```python
from build123d import *

# Parameters (mm, degrees)
SKETCH1_W           = 38
SKETCH1_H           = 53
SKETCH1_W_2         = 22
SKETCH1_H_2         = 42
BOSS_EXTRUDE1_DEPTH = 20
SKETCH2_W           = 8
SKETCH2_H           = 20
BOSS_EXTRUDE2_DEPTH = 20
SKETCH3_R           = 2.75
SKETCH3_R_2         = 1.6
CUT_EXTRUDE1_DEPTH  = 3
SKETCH3_2_R         = 1.6
CUT_EXTRUDE2_DEPTH  = 57.588426379
SKETCH4_R           = 1.6
CUT_EXTRUDE3_DEPTH  = 52.606685613
BOSS_EXTRUDE3_DEPTH = 8
FILLET2_R           = 3
FILLET1_R           = 5


with BuildPart() as part:
    # Sketch1 → Boss-Extrude1 (new body)
    with BuildSketch(Plane.XY):
        Rectangle(SKETCH1_W, SKETCH1_H)
        Rectangle(SKETCH1_W_2, SKETCH1_H_2, mode=Mode.SUBTRACT)
    extrude(amount=BOSS_EXTRUDE1_DEPTH)

    # Sketch2 → Boss-Extrude2 (add)
    with BuildSketch(Plane.XY.offset(20)):
        with Locations((-15, 11.5)):
            Rectangle(SKETCH2_W, SKETCH2_H)
    extrude(amount=BOSS_EXTRUDE2_DEPTH)

    # Sketch3 → Cut-Extrude1 (cut)
    # profile 1 of 2: a face of its own
    with BuildSketch(Plane(origin=(-11, 0, 0), x_dir=(0, 0, -1), z_dir=(1, 0, 0))):
        with Locations((-36, 11.5)):
            Circle(SKETCH3_R)
        with Locations((-36, 11.5)):
            Circle(SKETCH3_R_2, mode=Mode.SUBTRACT)
    # profile 2 of 2: a face of its own
    with BuildSketch(Plane(origin=(-11, 0, 0), x_dir=(0, 0, -1), z_dir=(1, 0, 0))):
        with Locations((-28, 11.5)):
            Circle(SKETCH3_R)
        with Locations((-28, 11.5)):
            Circle(SKETCH3_R_2, mode=Mode.SUBTRACT)
    extrude(amount=-CUT_EXTRUDE1_DEPTH, mode=Mode.SUBTRACT)

    # Sketch3<2> → Cut-Extrude2 (cut, through all)
    with BuildSketch(Plane(origin=(-11, 0, 0), x_dir=(0, 0, -1), z_dir=(1, 0, 0))):
        with Locations((-36, 11.5)):
            Circle(SKETCH3_2_R)
        with Locations((-28, 11.5)):
            Circle(SKETCH3_2_R)
    extrude(amount=-CUT_EXTRUDE2_DEPTH, mode=Mode.SUBTRACT)

    # Sketch4 → Cut-Extrude3 (cut, through all)
    with BuildSketch(Plane(origin=(0, 0, 0), x_dir=(-1, 0, 0), z_dir=(0, 0, -1))):
        with Locations((-5.1, -23.9)):
            Circle(SKETCH4_R)
        with Locations((5.1, -23.9)):
            Circle(SKETCH4_R)
        with Locations((-5.1, 23.9)):
            Circle(SKETCH4_R)
        with Locations((5.1, 23.9)):
            Circle(SKETCH4_R)
    extrude(amount=-CUT_EXTRUDE3_DEPTH, mode=Mode.SUBTRACT)

    # Sketch5 → Boss-Extrude3 (add)
    with BuildSketch(Plane.ZY.offset(19)):
        Polygon((32, 1.5), (20, -3.5), (20, 1.5), align=None)
        Polygon((20, 26.5), (20, 21.5), (32, 21.5), align=None)
    extrude(amount=-BOSS_EXTRUDE3_DEPTH)

    # Fillet2
    fillet2_edges = [part.edges().sort_by_distance(p)[0] for p in [
        (-15, 21.5, 32),
        (-15, 1.5, 40),
        (-15, 21.5, 40),
        (-15, -3.5, 20),
        (-15, 1.5, 32),
    ]]
    fillet(fillet2_edges, radius=FILLET2_R)

    # Fillet1
    fillet1_edges = [part.edges().sort_by_distance(p)[0] for p in [
        (-19, -26.5, 10),
        (19, -26.5, 10),
        (-19, 26.5, 10),
        (19, 26.5, 10),
    ]]
    fillet(fillet1_edges, radius=FILLET1_R - 0.0001)  # a hair under: the kernel refuses the full size


solid = part.part
```
Could you check a few things on this model? Use its own coordinates, in mm. A direction names the side the tool comes from. Round coordinates to 2 decimals unless told otherwise and drop trailing zeros. Write each loop counter-clockwise with the first axis right and the second up, starting at its lowest first coordinate (ties: lowest second). Pieces come first, ordered by that corner, then holes. Notation, with made-up numbers: M -37.5,-39 L 10.5,-39 A24 ccw 10.5,-15 Z; hole C 57,52.25 d3. An arc over 180 degrees is marked long. Write each question's results on one line, items separated by ' | '. Start each with the question number.
1. Imagine slicing it at D-D on z = 36. List the corners of the cut face in (x, y) for me, and give its area (4 significant figures).
2. I need wall thicknesses on L1, parallel to Y at x = -5.1, z = 6; L2, parallel to Z at x = -16, y = 11; L3, parallel to X at y = 23, z = 8. Which ranges of each line are inside material? Lowest first, please. Write a range as from..to.
3. Imagine slicing it at C-C on x = -9. List the corners of the cut face in (y, z) for me, and give its area (3 significant figures).
4. Thinking about a two-plate mould opening in X: for faces 1 (the face through (-17.57, 25, 12.9)), 2 (the face through (-11, 3, 16)), 3 (the face through (19, 0, 10)), which applies, +X half, -X half, draft (parallel to the pull), parting line (faces both ways), or undercut?
5. I'm going to push flat-ended pins straight in: pin 1 Ø1.3 at (x, z) = (-15.5, 34) entering from -Y; pin 2 Ø5 at (x, z) = (-14, 34.5) entering from +Y; pin 3 Ø5 at (y, z) = (11.5, 28) entering from +X. Where does each tip first touch, or does it pass through?
6. On a 3-axis mill with a long thin cutter (end or side, diameter ignored), from which of +Z, -Z, +X, -X, +Y, -Y can I reach the whole of each face in a straight line? I mean faces 4 (the face through (0, 21, 10)), 5 (the face through (-15, 21.5, 35)), 6 (the face through (-16.46, 12.58, 29.18)), 7 (the face through (-14, 10, 27)). Say none if no direction works.
7. Imagine slicing it at B-B on y = -17.5. List the corners of the cut face in (x, z) for me.
8. Imagine slicing it at A-A on x = -5.1. List the corners of the cut face in (y, z) for me, and give its area (3 significant figures).
Result sheet:
1) outline: M -19,1.5 L -11,1.5 L -11,8.75 L -14,8.75 L -14,9.9 L -19,9.9 Z; M -19,13.1 L -14,13.1 L -14,14.25 L -11,14.25 L -11,21.5 L -19,21.5 Z | area: 127.5 mm^2
2) L1: y = -26.5..-25.5, -22.3..-21, 21..22.3, 25.5..26.5 | L2: z = 0..26.48, 29.52..34.48, 37.52..40 | L3: x = -18.77..-6.42, -3.78..3.78, 6.42..18.77
3) outline: M -26.5,0 L -21,0 L -21,20 L -26.5,20 Z; M 21,0 L 26.5,0 L 26.5,20 L 21,20 Z | area: 220 mm^2
4) face 1: -X half | face 2: undercut | face 3: +X half
5) pin 1: stops at y = 1.5 | pin 2: stops at y = 21.56 | pin 3: stops at x = -14
6) face 4: +Z, -Z | face 5: +Z, +X, -X, +Y | face 6: +X, -X | face 7: +X
7) outline: M -19,0 L -11,0 L -11,20 L -19,20 Z; M 11,0 L 19,0 L 19,20 L 11,20 Z
8) outline: M -26.5,0 L -25.5,0 L -25.5,20 L -26.5,20 Z; M -22.3,0 L -21,0 L -21,20 L -22.3,20 Z; M 21,0 L 22.3,0 L 22.3,20 L 21,20 Z; M 25.5,0 L 26.5,0 L 26.5,20 L 25.5,20 Z | area: 92.0 mm^2
